CAD build for the part. Positions are in the model's coordinates, mm. Face numbers are marked on the shaded views. Round coordinates to 2 decimals unless told otherwise and drop trailing zeros. Loops run counter-clockwise (first coordinate to the right, second up) from the corner with the lowest first, then second, coordinate; pieces in that order, holes last. Notation, with made-up numbers: M -17.5,71.25 L -11.5,71.25 A19 ccw -11.5,76.25 Z; hole C 17.25,-37.5 d9. An arc over 180 degrees is marked long. Use a Markdown table: item, result. Add a question column.
(1) Band-saw the part on D-D, the plane z = 37. Write the cut outline in (x, y).
(2) Wall check: L1, parallel to X at y = -64.25, z = 10; L2, parallel to Y at x = 10, z = 11; L3, parallel to X at y = -24.5, z = 29.5. Give the ranges that are in metal, low to high.
(3) Band-saw the part on C-C, the plane z = 27. Write the cut outline in (x, y).
(4) Band-saw the part on B-B, the plane z = 16. Write the cut outline in (x, y).
(5) Flat gauge pins, fed straight in: P1, Ø6.5, axis at x = 10, y = -10, coming from the -Z side; P2, Ø7, axis at x = 70, y = -10, coming from the -Z side; P3, Ø5, axis at x = 70, y = -70, coming from the -Z side. Where does each tip first touch, or does it go through?
(6) Band-saw the part on A-A, the plane y = -54. Write the cut outline in (x, z), and give its area (3 significant figures).
(7) Two-plate mould, pull along Z, no slides. Class the marked faces 1, 2 and 3: released by +Z, released by -Z, zero draft, split by the parting line, or undercut.
from build123d import *

# Parameters (mm, degrees)
F0_W     = 80
F0_H     = 60
F0_R     = 16
F1_DEPTH = 80
F2_SIZE  = 7
F4_D     = 6
F4_DEPTH = 20
F4_TIP   = 1.8025818571
F6_D     = 8
F6_DEPTH = 20
F6_TIP   = 2.4034424761


with BuildPart() as f1:
    # F0 (on Front) → F1 (new body)
    with BuildSketch(Plane.XZ):
        with Locations((40, 30)):
            Rectangle(F0_W, F0_H)
        with Locations((40, 30)):
            Circle(F0_R, mode=Mode.SUBTRACT)
    extrude(amount=F1_DEPTH)

    # F2
    f2_edges = [f1.edges().sort_by_distance(p)[0] for p in [
        (0, -40, 60),
        (80, -40, 60),
    ]]
    chamfer(f2_edges, length=F2_SIZE)

    # F4
    with Locations(Plane.XZ.offset(80)):
        with Locations((20, 50), (60, 50), (60, 10), (20, 10)):
            Hole(F4_D / 2, depth=F4_DEPTH)
            with Locations((0, 0, -(F4_DEPTH + F4_TIP / 2))):  # 118° drill point
                Cone(0, F4_D / 2, F4_TIP, mode=Mode.SUBTRACT)

    # F6
    with Locations(Plane(origin=(0, 0, 0), x_dir=(1, 0, 0), z_dir=(0, 0, -1))):
        with Locations((10, 70), (70, 70), (70, 10), (10, 10)):
            Hole(F6_D / 2, depth=F6_DEPTH)
            with Locations((0, 0, -(F6_DEPTH + F6_TIP / 2))):  # 118° drill point
                Cone(0, F6_D / 2, F6_TIP, mode=Mode.SUBTRACT)


solid = f1.part
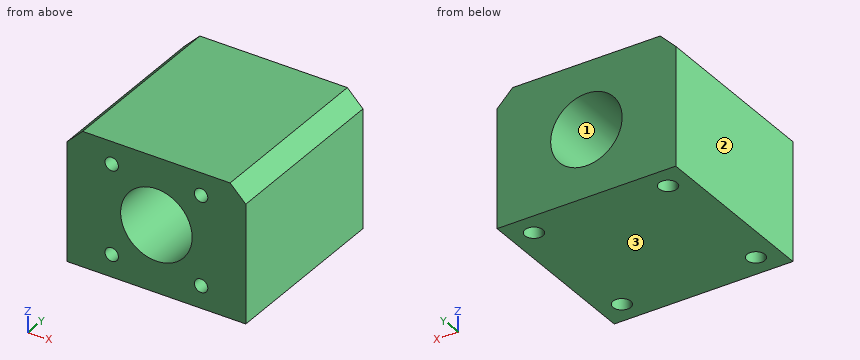
Return value:
| question | item | result |
|---|---|---|
| 1 | outline | M 0,-80 L 25.61,-80 L 25.61,0 L 0,0 Z; M 54.39,-80 L 80,-80 L 80,0 L 54.39,0 Z |
| 2 | L1 | 0 to 17, 23 to 57, 63 to 80 |
| 2 | L2 | -80 to -74, -66 to -14, -6 to 0 |
| 2 | L3 | 0 to 24.01, 55.99 to 80 |
| 3 | outline | M 0,-80 L 24.28,-80 L 24.28,0 L 0,0 Z; M 55.72,-80 L 80,-80 L 80,0 L 55.72,0 Z |
| 4 | outline | M 0,-80 L 32.25,-80 L 32.25,0 L 0,0 Z; M 47.75,-80 L 80,-80 L 80,0 L 47.75,0 Z; hole C 10,-70 d8; hole C 10,-10 d8; hole C 70,-70 d8; hole C 70,-10 d8 |
| 5 | P1 | z = 20.45 |
| 5 | P2 | z = 20.3 |
| 5 | P3 | z = 20.9 |
| 6 | outline | M 0,0 L 80,0 L 80,53 L 73,60 L 7,60 L 0,53 Z; hole C 40,30 d32 |
| 6 | area | 3,950 mm^2 |
| 7 | face 1 | undercut |
| 7 | face 2 | zero draft |
| 7 | face 3 | released by -Z |
